Check sheet for the modelled part. Datum: model origin and axes. Units: mm. Coordinates: 2 decimals unless noted, no trailing zeros. Loops run counter-clockwise (first coordinate to the right, second up) from the corner with the lowest first, then second, coordinate; pieces in that order, holes last. Notation, with made-up numbers: M -36.75,13 L -27.75,13 A23 ccw -27.75,38 Z; hole C 29,20 d9. An arc over 180 degrees is marked long. Answer in a Markdown table with one row per item. Add a question column.
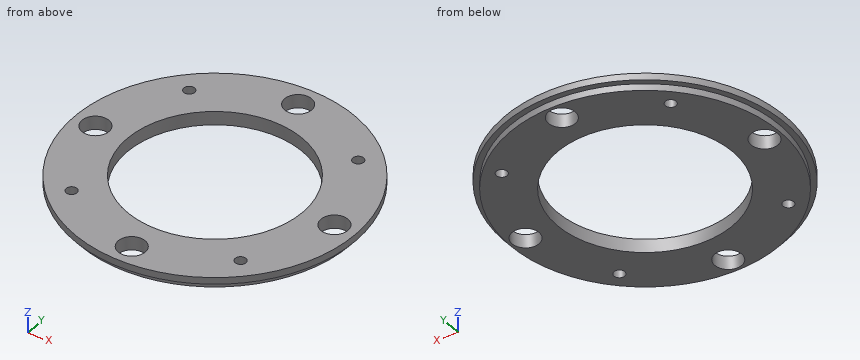
Autodesk Inventor part; units mm, degrees
ref_plane "YZ Plane" through (0, 0, 0) normal (1, 0, 0) x (0, 1, 0)
ref_plane "XZ Plane" through (0, 0, 0) normal (0, 1, 0) x (-1, 0, 0)
ref_plane "XY Plane" through (0, 0, 0) normal (0, 0, 1) x (1, 0, 0)
sketch "スケッチ1" plane through (0, 0, 0) normal (0, 0, 1) x (1, 0, 0)
  circle A0 centre (0, 0) radius 50
  dimension "d0" = 100
extrude "押し出し1" add sketch "スケッチ1" along normal blind 2.5
sketch "スケッチ2" plane through (0, 0, 2.5) normal (0, 0, 1) x (1, 0, 0)
  circle A0 centre (0, 0) radius 52
  dimension "d3" = 104
extrude "押し出し2" add sketch "スケッチ2" along normal blind 2.5
sketch "スケッチ3" plane through (0, 0, 5) normal (0, 0, 1) x (1, 0, 0)
  point P0 (0, 0)
  point P1 (0, 44)
  dimension "d6" = 44
hole "穴1" at (0, 44, 5) direction (0, 0, -1) diameter 10 end through all
pattern_circular "円形状パターン1" count 4 over 360 about axis through (0, 0, 0) along (0, 0, 1) of "穴1"
sketch "スケッチ4" plane through (0, 0, 5) normal (0, 0, 1) x (1, 0, 0)
  circle A0 centre (0, -44) radius 5
  circle A1 centre (0, 0) radius 44
  line L0 (0, 0) -> (31.1127, 31.1127)
  arc A2 (0, 3.9955) -> (0, 0) centre (1.9978, 1.9978) ccw
  line L1 (0, 3.9955) -> (0, 44)
  dimension "d17" = 45
hole "穴2" at (31.1127, 31.1127, 5) direction (0, 0, -1) diameter 4 end through all
thread "ねじ1"
pattern_circular "円形状パターン2" count 4 over 360 about axis through (0, 0, 0) along (0, 0, 1) of "穴2"
sketch "スケッチ5" plane through (0, 0, 5) normal (0, 0, 1) x (1, 0, 0)
  circle A0 centre (0, 0) radius 32.5
  dimension "d30" = 65
extrude "押し出し3" cut sketch "スケッチ5" against normal through all
properties part number "出力板表" material "アルミニウム 6061"
Q1. Cross-section at C-C (y = -44). Record the cut outline in (x, z).
Q2. Thickness scan on L1, parallel to Y at x = -4, z = 3.25; L2, parallel to X at y = 3, z = 3.65; L3, parallel to X at y = -24, z = 1.9. Record the ranges inside material, lowest first.
Q3. Cross-section at A-A (y = 0). Record the cut outline in (x, z).
Q4. Cross-section at D-D (x = -41). Record the cut outline in (y, z), plus the area to 3 significant figures.
Q5. Go/stop test with flat-tipped pins: pin 1 (2 mm diameter, centred on x = 25, y = -26.5, fed in from -Z); pin 2 (1 mm diameter, centred on y = -38.5, z = 3.5, fed in from -X); pin 3 (3 mm diameter, centred on y = 11, z = 2.5, fed in from -X). Record where each tip stops, or that it passes through.
Answer key:
| question | item | result |
|---|---|---|
| 1 | outline | M -27.71,2.5 L -23.75,2.5 L -23.75,0 L -5,0 L -5,5 L -27.71,5 Z; M 5,0 L 23.75,0 L 23.75,2.5 L 27.71,2.5 L 27.71,5 L 5,5 Z |
| 2 | L1 | -51.85 to -47, -41 to -32.25, 32.25 to 41, 47 to 51.85 |
| 2 | L2 | -51.91 to -48, -40 to -32.36, 32.36 to 40, 48 to 51.91 |
| 2 | L3 | -43.86 to -21.91, 21.91 to 43.86 |
| 3 | outline | M -52,2.5 L -50,2.5 L -50,0 L -49,0 L -49,5 L -52,5 Z; M -39,0 L -32.5,0 L -32.5,5 L -39,5 Z; M 32.5,0 L 39,0 L 39,5 L 32.5,5 Z; M 49,0 L 50,0 L 50,2.5 L 52,2.5 L 52,5 L 49,5 Z |
| 4 | outline | M -31.98,2.5 L -28.62,2.5 L -28.62,0 L -4,0 L -4,5 L -31.98,5 Z; M 4,0 L 28.62,0 L 28.62,2.5 L 31.98,2.5 L 31.98,5 L 4,5 Z |
| 4 | area | 263 mm^2 |
| 5 | pin 1 | z = 0 |
| 5 | pin 2 | x = -35.5 |
| 5 | pin 3 | x = -51.12 |
